Part model, mm, in its own coordinate system. A direction names the side the tool comes from. Give positions to 0.01 mm unless a question says otherwise; leave off trailing zeros. Write each loop counter-clockwise with the first axis right and the second up, starting at its lowest first coordinate (ties: lowest second). Pieces come first, ordered by that corner, then holes. Notation, with made-up numbers: (-19, -25.75) - (23, -25.75) arc R18 ccw to (23, -14.75) - close; hole circle Ø7 at (11, 8). An arc over 180 degrees is marked (long way). Answer in a Markdown table with one row per item. Add a question column.
1. Which spindle directions (+Z, -Z, +X, -X, +Y, -Y) get a long thin tool onto all of the face, cutting with end or side? Do faces 1 (the flat face through (-4, 1.143, -1)), 2 (the flat face through (4, -1.143, -1)). Say none if no direction does.
2. Band-saw the part on D-D on z = 46.5. Write the cut outline in (x, y).
3. Drop flat-ended pins along their axis: pin 1 Ø0.7 at (x, y) = (315.5, 0) entering from +Z; pin 2 Ø8 at (x, z) = (4, 56) entering from +Y; pin 3 Ø0.5 at (x, y) = (-138, 1.5) entering from +Z. Give the stop position or say it passes through.
4. Band-saw the part on B-B on x = 212.5. Write the cut outline in (y, z).
5. Probe line 1 along X through (y, z) = (-0.05, -60); line 2 along Y through (x, z) = (-45.5, -10.5); line 3 along X through (y, z) = (-1, 53). List the from-to ranges inside material, lowest first.
6. Band-saw the part on A-A on z = -43.5. Write the cut outline in (x, y).
7. Band-saw the part on C-C on z = 10. Write the cut outline in (x, y).
```python
from build123d import *

# Parameters (mm, degrees)
SKETCH1_W           = 635.3556
SKETCH1_H           = 145.542
BOSS_EXTRUDE1_DEPTH = 1.143
SKETCH2_W           = 254
SKETCH2_H           = 2.7305
BOSS_EXTRUDE2_DEPTH = 3.175
SKETCH3_W           = 3.175
SKETCH3_H           = 38.1
CUT_EXTRUDE1_DEPTH  = 3.7305
SKETCH4_W           = 2.286
SKETCH4_H           = 72.771
CUT_EXTRUDE2_DEPTH  = 3.7305


with BuildPart() as part:
    # Sketch1 → Boss-Extrude1 (new body, symmetric)
    with BuildSketch(Plane(origin=(0, 0, 0), x_dir=(1, 0, 0), z_dir=(0, 1, 0))):
        Rectangle(SKETCH1_W, SKETCH1_H)
    extrude(amount=BOSS_EXTRUDE1_DEPTH, both=True)

    # Sketch2 → Boss-Extrude2 (add)
    with BuildSketch(Plane(origin=(0, 0, -72.771), x_dir=(-1, 0, 0), z_dir=(0, 0, -1))):
        with Locations((-157.8229, 0.22225)):
            Rectangle(SKETCH2_W, SKETCH2_H)
        with Locations((157.8229, 0.22225)):
            Rectangle(SKETCH2_W, SKETCH2_H)
    extrude(amount=BOSS_EXTRUDE2_DEPTH)

    # Sketch3 → Cut-Extrude1 (cut, through all)
    with BuildSketch(Plane.XZ.offset(1.143)):
        with Locations((-316.0903, 53.721)):
            Rectangle(SKETCH3_W, SKETCH3_H)
    cut_extrude1 = extrude(amount=-CUT_EXTRUDE1_DEPTH, mode=Mode.SUBTRACT)

    # Mirror1: Cut-Extrude1 across plane
    add(cut_extrude1.mirror(Plane(origin=(0, 0, 0), x_dir=(0, 0, 1), z_dir=(1, 0, 0))), mode=Mode.SUBTRACT)

    # Sketch4 → Cut-Extrude2 (cut, through all)
    with BuildSketch(Plane.XZ.offset(1.143)):
        with Locations((0, -36.3855)):
            Rectangle(SKETCH4_W, SKETCH4_H)
    extrude(amount=-CUT_EXTRUDE2_DEPTH, mode=Mode.SUBTRACT)


solid = part.part
```
Values:
| question | item | result |
|---|---|---|
| 1 | face 1 | +Z, +X, -X, +Y |
| 1 | face 2 | +Z, -Z, +X, -X, -Y |
| 2 | outline | (-314.5, -1.14) - (314.5, -1.14) - (314.5, 1.14) - (-314.5, 1.14) - close |
| 3 | pin 1 | stops at z = 34.67 |
| 3 | pin 2 | stops at y = 1.14 |
| 3 | pin 3 | stops at z = -72.77 |
| 4 | outline | (-1.14, -75.95) - (1.59, -75.95) - (1.59, -72.77) - (1.14, -72.77) - (1.14, 72.77) - (-1.14, 72.77) - close |
| 5 | line 1 | x = -317.68 to -1.14, 1.14 to 317.68 |
| 5 | line 2 | y = -1.14 to 1.14 |
| 5 | line 3 | x = -314.5 to 314.5 |
| 6 | outline | (-317.68, -1.14) - (-1.14, -1.14) - (-1.14, 1.14) - (-317.68, 1.14) - close; (1.14, -1.14) - (317.68, -1.14) - (317.68, 1.14) - (1.14, 1.14) - close |
| 7 | outline | (-317.68, -1.14) - (317.68, -1.14) - (317.68, 1.14) - (-317.68, 1.14) - close |
